```python
from build123d import *

# Parameters (mm, degrees)
SKETCH1_W                 = 50
SKETCH1_H                 = 95
BOSS_EXTRUDE1_DEPTH       = 6.35
M4X0_7_TAPPED_HOLE1_D     = 3.3
M4X0_7_TAPPED_HOLE1_DEPTH = 10
M4X0_7_TAPPED_HOLE1_TIP   = 0.991420021
M4X0_7_TAPPED_HOLE2_D     = 3.3
M4X0_7_TAPPED_HOLE2_DEPTH = 10
M4X0_7_TAPPED_HOLE2_TIP   = 0.991420021
SKETCH7_R                 = 11.3175
CUT_EXTRUDE1_DEPTH        = 55.051572595
M3_CLEARANCE_HOLE1_D      = 3.6


with BuildPart() as part:
    # Sketch1 → Boss-Extrude1 (new body)
    with BuildSketch(Plane.XY):
        Rectangle(SKETCH1_W, SKETCH1_H)
    extrude(amount=-BOSS_EXTRUDE1_DEPTH)

    # M4x0.7 Tapped Hole1
    with Locations(Plane.XZ.offset(47.5)):
        with Locations((-16.67, -3.175), (16.67, -3.175), (0, -3.175)):
            Hole(M4X0_7_TAPPED_HOLE1_D / 2, depth=M4X0_7_TAPPED_HOLE1_DEPTH)
            with Locations((0, 0, -(M4X0_7_TAPPED_HOLE1_DEPTH + M4X0_7_TAPPED_HOLE1_TIP / 2))):  # 118° drill point
                Cone(0, M4X0_7_TAPPED_HOLE1_D / 2, M4X0_7_TAPPED_HOLE1_TIP, mode=Mode.SUBTRACT)

    # M4x0.7 Tapped Hole2
    with Locations(Plane(origin=(0, 47.5, 0), x_dir=(1, 0, 0), z_dir=(0, 1, 0))):
        with Locations((-16.67, 3.175), (0, 3.175), (16.67, 3.175)):
            Hole(M4X0_7_TAPPED_HOLE2_D / 2, depth=M4X0_7_TAPPED_HOLE2_DEPTH)
            with Locations((0, 0, -(M4X0_7_TAPPED_HOLE2_DEPTH + M4X0_7_TAPPED_HOLE2_TIP / 2))):  # 118° drill point
                Cone(0, M4X0_7_TAPPED_HOLE2_D / 2, M4X0_7_TAPPED_HOLE2_TIP, mode=Mode.SUBTRACT)

    # Sketch7 → Cut-Extrude1 (cut, through all)
    with BuildSketch(Plane(origin=(0, 0, -6.35), x_dir=(-1, 0, 0), z_dir=(0, 0, -1))):
        Circle(SKETCH7_R)
    extrude(amount=-CUT_EXTRUDE1_DEPTH, mode=Mode.SUBTRACT)

    # M3 Clearance Hole1 (through all)
    with Locations(Plane(origin=(0, 0, -6.35), x_dir=(-1, 0, 0), z_dir=(0, 0, -1))):
        with Locations((-9.899494937, 9.899494937), (9.899494937, 9.899494937), (9.899494937, -9.899494937), (-9.899494937, -9.899494937), (0, 0)):
            Hole(M3_CLEARANCE_HOLE1_D / 2)


solid = part.part
```
Source: CAD feature listing. Evaluate the final solid. Frame: model axes, mm. A direction names the side the tool comes from. Round coordinates to 2 decimals unless told otherwise and drop trailing zeros. Loops run counter-clockwise (first coordinate to the right, second up) from the corner with the lowest first, then second, coordinate; pieces in that order, holes last.
(1) Access query for faces 1 (the cylindrical face through (18.32, -42.43, -3.1)), 2 (the cylindrical face through (-17.43, 42.43, -1.71)), 3 (the cylindrical face through (11.616, 10.44, -3.131)). Directions: +Z, -Z, +X, -X, +Y, -Y. A direction counts if a zero-diameter tool reaches every point of the face in a straight line with its end or side. Return the directions, or none.
From the geometry:
face 1: -Y
face 2: +Y
face 3: +Z, -Z
(2) Material intervals for probe 1 along X at (y, z) = (38.5, -1.75); probe 2 along Z at (x, y) = (0, -44.5) (3 decimals); probe 3 along X at (y, z) = (10, -0.25), sorted ascending.
From the geometry:
probe 1: x = -25 to -17.5, -15.84 to -0.83, 0.83 to 15.84, 17.5 to 25
probe 2: z = -6.35 to -4.825, -1.525 to 0
probe 3: x = -25 to -11.7, -8.1 to -5.3, 5.3 to 8.1, 11.7 to 25
(3) Section query A-A (y = 0). Output: boundary loops of the cut face in (x, z), and give its area (3 significant figures).
From the geometry:
outline: (-25, -6.35) - (-11.32, -6.35) - (-11.32, 0) - (-25, 0) - close; (11.32, -6.35) - (25, -6.35) - (25, 0) - (11.32, 0) - close
area: 174 mm2
(4) Section query B-B (x = -5.5). Output: boundary loops of the cut face in (y, z), and give its area (3 significant figures).
From the geometry:
outline: (-47.5, -6.35) - (-9.89, -6.35) - (-9.89, 0) - (-47.5, 0) - close; (9.89, -6.35) - (47.5, -6.35) - (47.5, 0) - (9.89, 0) - close
area: 478 mm2
(5) Contact query for flat-ended pins moving along their axis: pin 1 Ø3 at (x, y) = (-9.9, 9.9) entering from +Z; pin 2 Ø2 at (x, z) = (-16.67, -3.175) entering from +Y; pin 3 Ø2 at (x, z) = (-16.67, -3.175) entering from -Y. Output: stop coordinate, or through.
From the geometry:
pin 1: passes through
pin 2: stops at y = 37.11
pin 3: stops at y = -37.11
(6) Pull-direction query (Y, two-part tool) for faces 4 (the cylindrical face through (-8.183, -9.359, -3.131)), 5 (the cylindrical face through (11.616, -9.359, -3.131)), 6 (the cylindrical face through (-17.43, -42.43, -4.64)), 7 (the flat face through (0, -47.5, -5)); classes: +Y half, -Y half, draft (parallel to the pull), parting line (faces both ways), or undercut.
From the geometry:
face 4: undercut
face 5: undercut
face 6: draft
face 7: -Y half
